from build123d import *

# Parameters (mm, degrees)
F0_R      = 9.3155
F1_DEPTH  = 11
F2_R      = 12
F2_R_2    = 10.5
F3_DEPTH  = 20
F4_R      = 9.3155
F5_DEPTH  = 11
F6_R      = 12
F7_DEPTH  = 25
F9_DEPTH  = 10
F10_R     = 4
F11_DEPTH = 73
F12_W     = 18.0728212726
F12_H     = 3
F12_W_2   = 18.3906073943
F12_W_3   = 3
F12_H_2   = 17.3976836615
F12_H_3   = 17.163570568
F13_DEPTH = 5
F14_R     = 25
F14_R_2   = 19.9436706752
F15_DEPTH = 5


with BuildPart() as f1:
    # F0 (on Front) → F1 (new body)
    with BuildSketch(Plane.XZ):
        Polygon((13, -5.3847763109), (13, 5.3847763109), (5.3847763109, 13), (-5.3847763109, 13), (-13, 5.3847763109), (-13, -5.3847763109), (-5.3847763109, -13), (5.3847763109, -13), align=None)
        Circle(F0_R, mode=Mode.SUBTRACT)
    extrude(amount=F1_DEPTH)

    # F2 (on face) → F3 (join)
    with BuildSketch(Plane(origin=(0, 0, 0), x_dir=(-1, 0, 0), z_dir=(0, 1, 0))):
        Circle(F2_R)
        Circle(F2_R_2, mode=Mode.SUBTRACT)
    extrude(amount=F3_DEPTH)

    # F4 (on face) → F5 (join)
    with BuildSketch(Plane(origin=(0, 20, 0), x_dir=(-1, 0, 0), z_dir=(0, 1, 0))):
        Polygon((13, -5.3847763109), (13, 5.3847763109), (5.3847763109, 13), (-5.3847763109, 13), (-13, 5.3847763109), (-13, -5.3847763109), (-5.3847763109, -13), (5.3847763109, -13), align=None)
        Circle(F4_R, mode=Mode.SUBTRACT)
    extrude(amount=F5_DEPTH)

    # F6 (on Top) → F7 (join)
    with BuildSketch(Plane.XY):
        with Locations((0, 10.1140267726)):
            Circle(F6_R)
    extrude(amount=F7_DEPTH)

    # F8 (on face) → F9 (join)
    with BuildSketch(Plane.XY.offset(25)):
        Polygon((-3.2036065086, 4.5652175322), (3.2036065086, 4.5652175322), (6.4072130172, 10.1140267726), (3.2036065086, 15.6628360129), (-3.2036065086, 15.6628360129), (-6.4072130172, 10.1140267726), align=None)
    extrude(amount=F9_DEPTH)

    # F10 (on Top) → F11 (join)
    with BuildSketch(Plane.XY):
        with Locations((0, 10)):
            Circle(F10_R)
    extrude(amount=F11_DEPTH)

    # F12 (on face) → F13 (join)
    with BuildSketch(Plane.XY.offset(73)):
        with Locations((-10.9072600389, 10)):
            Rectangle(F12_W, F12_H)
        with Locations((10.748366978, 10)):
            Rectangle(F12_W_2, F12_H)
        with Locations((0, -1.2448288445)):
            Rectangle(F12_W_3, F12_H_2)
        with Locations((0, 21.3618853912)):
            Rectangle(F12_W_3, F12_H_3)
    extrude(amount=-F13_DEPTH)

    # F14 (on face) → F15 (join)
    with BuildSketch(Plane.XY.offset(73)):
        with Locations((0, 10)):
            Circle(F14_R)
        with Locations((0, 10)):
            Circle(F14_R_2, mode=Mode.SUBTRACT)
    extrude(amount=-F15_DEPTH)


solid = f1.part
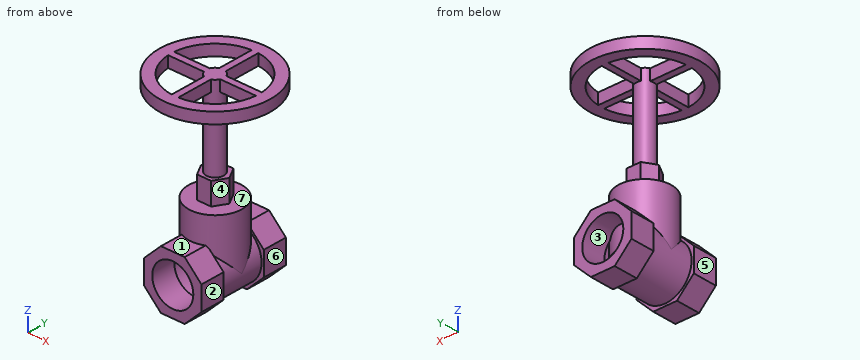
Read the model definition and answer for the solid it produces. Units are mm, in the model's axes. Face numbers are marked on the shaded views. A direction names the side the tool comes from. Round coordinates to 2 decimals unless told otherwise and drop trailing zeros. Order: outer loops, then holes, each group sorted by start corner. A loop starts at its lowest first (then second) coordinate and runs counter-clockwise, first axis right, second up. Notation, with made-up numbers: (86, 56.25) - (106, 56.25) arc R18 ccw to (106, 68.25) - close; hole circle Ø5 at (75.5, 2). An arc over 180 degrees is marked (long way). Use one line per item in the form item = value. Start each with the question number.
(1) Flat-ended cylindrical pins translate along their axes: pin 1 Ø1.5 at (x, z) = (10.5, 71) entering from -Y; pin 2 Ø8 at (x, z) = (-1.5, 2.5) entering from +Y; pin 3 Ø6 at (x, z) = (6, 52.5) entering from -Y. Find the tip coordinate at first contact, or state that the pin passes through.
(2) Determine the mould class of the marked faces 1, 2 and 3 for opening direction X: +X half, -X half, draft (parallel to the pull), parting line (faces both ways), or undercut.
(3) Find the intervals of material crossed by line 1 along Z through (x, y) = (-0.5, 17.5); line 2 along Z through (x, y) = (0, 24.75); line 3 along X through (y, z) = (23, 0), in increasing order. Write a range as from..to.
(4) The part is cut by section D-D (z = 15). Give the vertices of the cut face in (x, y), then the cut area to 3 significant figures.
(5) The part is cut by section B-B (x = 17.5). Give the vertices of the cut face in (y, z).
(6) The part is cut by section A-A (y = -6.5). Give the vertices of the cut face in (x, z), then the cut area to 3 significant figures.
(7) For the marked faces 4, 5, 6 and 7, determine the directions among +Z, -Z, +X, -X, +Y, -Y from which every point of the face is accessible in a straight line to the end or side of a thin tool.
(8) The part is cut by section C-C (y = 3). Give the vertices of the cut face in (x, z).
Checked values:
q1.pin_1 = -13.02
q1.pin_2 = 22.11
q1.pin_3 = 7.35
q2.face_1 = draft
q2.face_2 = +X half
q2.face_3 = undercut
q3.line_1 = -11.99..-10.49, 0..25, 68..73
q3.line_2 = -13..-9.32, 9.32..13, 68..73
q3.line_3 = -13..-9.32, 9.32..13
q4.outline = circle Ø24 at (0, 10.11)
q4.area = 452 mm^2
q5.outline = (-7.85, 68) - (0.43, 68) - (0.43, 73) - (-7.85, 73) - close; (8.5, 68) - (11.5, 68) - (11.5, 73) - (8.5, 73) - close; (19.57, 68) - (27.85, 68) - (27.85, 73) - (19.57, 73) - close
q6.outline = (-18.78, 68) - (-11.2, 68) - (-11.2, 73) - (-18.78, 73) - close; (-13, -5.38) - (-5.38, -13) - (5.38, -13) - (13, -5.38) - (13, 5.38) - (5.38, 13) - (-5.38, 13) - (-13, 5.38) - close; (-1.5, 68) - (1.5, 68) - (1.5, 73) - (-1.5, 73) - close; (11.2, 68) - (18.78, 68) - (18.78, 73) - (11.2, 73) - close; hole circle Ø18.63 at (0, 0)
q6.area = 378 mm^2
q7.face_4 = +X, -Y
q7.face_5 = -Z, -X, +Y, -Y
q7.face_6 = -Z, +X, +Y, -Y
q7.face_7 = none
q8.outline = (-24, 68) - (-18.67, 68) - (-18.67, 73) - (-24, 73) - close; (-9.66, 7.11) arc R12 ccw (long way) to (9.66, 7.11) - (9.66, 25) - (-9.66, 25) - close; (-1.5, 68) - (1.5, 68) - (1.5, 73) - (-1.5, 73) - close; (18.67, 68) - (24, 68) - (24, 73) - (18.67, 73) - close; hole (-9.66, 0) - (-9.66, 4.11) arc R10.5 ccw (long way) to (9.66, 4.11) - (9.66, 0) - close
